from build123d import *

# Parameters (mm, degrees)
PAD_DEPTH             = 24
POCKET_DEPTH          = 3
SKETCH002_W           = 70
SKETCH002_H           = 18.5
POCKET001_DEPTH       = 18
POLARPATTERN_COUNT    = 3
POCKET002_DEPTH       = 6
CHAMFER_SIZE          = 8
FILLET_R              = 13
FILLET001_R           = 11
CHAMFER001_SIZE       = 16.1
FILLET002_R           = 11
FILLET003_R           = 12
POCKET003_DEPTH       = 6
POCKET004_DEPTH       = 18
POCKET005_DEPTH       = 21.001
SKETCH007_W           = 15.5
SKETCH007_H           = 15
POCKET006_DEPTH       = 5
SKETCH010_W           = 13.6
SKETCH010_H           = 9
POCKET009_DEPTH       = 15.5
POCKET010_DEPTH       = 3
SKETCH012_R           = 1.85
SKETCH012_R_2         = 0.99
POCKET011_DEPTH       = 498.0492855781
POLARPATTERN001_COUNT = 3
POCKET012_DEPTH       = 12


with BuildPart() as part:
    # Sketch → Pad (new body)
    with BuildSketch(Plane.XY):
        Polygon((0, 112.2094915052), (-97.1762701892, -56.1047457526), (97.1762701892, -56.1047457526), align=None)
        Polygon((0, 62.2094915052), (-53.875, -31.1047457526), (53.875, -31.1047457526), align=None, mode=Mode.SUBTRACT)
    extrude(amount=PAD_DEPTH)

    # Sketch001 (on Face8 of Pad) → Pocket (cut)
    with BuildSketch(Plane.XY.offset(24)):
        Polygon((0, 98.2094915052), (-85.0519145362, -49.1047457526), (85.0519145362, -49.1047457526), align=None)
        Polygon((0, 76.2094915052), (-65.999355653, -38.1047457526), (65.999355653, -38.1047457526), align=None, mode=Mode.SUBTRACT)
    extrude(amount=-POCKET_DEPTH, mode=Mode.SUBTRACT)

    # Sketch002 (on Face4 of Pocket) → Pocket001 (cut)
    with BuildSketch(Plane(origin=(0, 0, 0), x_dir=(1, 0, 0), z_dir=(0, 0, -1))):
        with Locations((0, 43.6047457526)):
            Rectangle(SKETCH002_W, SKETCH002_H)
    pocket001 = extrude(amount=-POCKET001_DEPTH, mode=Mode.SUBTRACT)

    # PolarPattern: Pocket001 ×3 about axis
    polarpattern_axis = Axis((0, 0, 0), (0, 0, -1))
    for i in range(1, POLARPATTERN_COUNT):
        add(pocket001.rotate(polarpattern_axis, i * 360 / POLARPATTERN_COUNT), mode=Mode.SUBTRACT)

    # Sketch003 (on Face4 of PolarPattern) → Pocket002 (cut)
    with BuildSketch(Plane(origin=(0, 0, 0), x_dir=(1, 0, 0), z_dir=(0, 0, -1))):
        Polygon((0, -100.2094915052), (86.7839653438, 50.1047457526), (-86.7839653438, 50.1047457526), align=None)
        Polygon((0, -74.2094915052), (64.2673048454, 37.1047457526), (-64.2673048454, 37.1047457526), align=None, mode=Mode.SUBTRACT)
    extrude(amount=-POCKET002_DEPTH, mode=Mode.SUBTRACT)

    # Chamfer
    chamfer_edges = [part.edges().sort_by_distance(p)[0] for p in [
        (-53.875, -31.104746, 12),
        (53.875, -31.104746, 12),
        (0, 62.209492, 12),
    ]]
    chamfer(chamfer_edges, length=CHAMFER_SIZE)

    # Fillet
    fillet_edges = [part.edges().sort_by_distance(p)[0] for p in [
        (0, 100.209492, 3),
        (-86.783965, -50.104746, 3),
        (86.783965, -50.104746, 3),
    ]]
    fillet(fillet_edges, radius=FILLET_R)

    # Fillet001
    fillet001_edges = [part.edges().sort_by_distance(p)[0] for p in [
        (0, 74.209492, 3),
        (64.267305, -37.104746, 3),
        (-64.267305, -37.104746, 3),
    ]]
    fillet(fillet001_edges, radius=FILLET001_R)

    # Chamfer001
    chamfer001_edges = [part.edges().sort_by_distance(p)[0] for p in [
        (97.17627, -56.104746, 12),
        (0, 112.209492, 12),
        (-97.17627, -56.104746, 12),
    ]]
    chamfer(chamfer001_edges, length=CHAMFER001_SIZE)

    # Fillet002
    fillet002_edges = [part.edges().sort_by_distance(p)[0] for p in [
        (0, 98.209492, 22.5),
        (-85.051915, -49.104746, 22.5),
        (85.051915, -49.104746, 22.5),
    ]]
    fillet(fillet002_edges, radius=FILLET002_R)

    # Fillet003
    fillet003_edges = [part.edges().sort_by_distance(p)[0] for p in [
        (65.999356, -38.104746, 22.5),
        (0, 76.209492, 22.5),
        (-65.999356, -38.104746, 22.5),
    ]]
    fillet(fillet003_edges, radius=FILLET003_R)

    # Sketch004 (on Face60 of Fillet003) → Pocket003 (cut)
    with BuildSketch(Plane(origin=(0, 0, 6), x_dir=(1, 0, 0), z_dir=(0, 0, -1))):
        Polygon((-8.75, -71.2664825043), (8.75, -71.2664825043), (8.75, -94.7664825043), (4, -94.7664825043), (4, -98.2664825043), (-4, -98.2664825043), (-4, -94.7664825043), (-8.75, -94.7664825043), align=None)
    extrude(amount=-POCKET003_DEPTH, mode=Mode.SUBTRACT)

    # Sketch005 (on Face29 of Pocket003) → Pocket004 (cut)
    with BuildSketch(Plane(origin=(0, 0, 0), x_dir=(1, 0, 0), z_dir=(0, 0, -1))):
        Polygon((46.1715988394, 38.9547457526), (68.6882593378, 51.9547457526), (79.3382593378, 33.508404652), (56.8215988394, 20.508404652), align=None)
    extrude(amount=-POCKET004_DEPTH, mode=Mode.SUBTRACT)

    # Sketch006 (on Face1 of Pocket004) → Pocket005 (cut, through all)
    with BuildSketch(Plane.XY.offset(21)):
        with BuildLine():
            ThreePointArc((1.5, 85.0404521425), (0, 86.5404521425), (-1.5, 85.0404521425))
            Line((-1.5, 85.0404521425), (-1.5, 66.0404521425))
            ThreePointArc((-1.5, 66.0404521425), (0, 64.5404521425), (1.5, 66.0404521425))
            Line((1.5, 85.0404521425), (1.5, 66.0404521425))
        make_face()
    extrude(amount=-POCKET005_DEPTH, mode=Mode.SUBTRACT)

    # Sketch007 (on Face24 of Pocket005) → Pocket006 (cut)
    with BuildSketch(Plane(origin=(-48.5881350946, 28.0523728763, 0), x_dir=(-0.5, -0.8660254038, 0), z_dir=(-0.8660254038, 0.5, 0))):
        with Locations((-47.3262701892, 13.5)):
            Rectangle(SKETCH007_W, SKETCH007_H)
    extrude(amount=-POCKET006_DEPTH, mode=Mode.SUBTRACT)

    # Sketch010 (on Face79 of Pocket006) → Pocket009 (cut)
    with BuildSketch(Plane(origin=(-44.2580080757, 25.5523728763, 0), x_dir=(-0.5, -0.8660254038, 0), z_dir=(-0.8660254038, 0.5, 0))):
        with Locations((-47.3262701892, 13.5)):
            Rectangle(SKETCH010_W, SKETCH010_H)
    extrude(amount=-POCKET009_DEPTH, mode=Mode.SUBTRACT)

    # Sketch011 (on Face21 of Pocket009) → Pocket010 (cut)
    with BuildSketch(Plane(origin=(0, 0, 6), x_dir=(1, 0, 0), z_dir=(0, 0, -1))):
        Polygon((-21.0413798427, -59.7570681827), (-11.6817654684, -54.3532923042), (-6.658482036, -63.0538744299), (-16.0180964103, -68.4576503084), align=None)
    extrude(amount=-POCKET010_DEPTH, mode=Mode.SUBTRACT)

    # Sketch012 (on Face54 of Pocket010) → Pocket011 (cut, through all)
    with BuildSketch(Plane(origin=(0, 0, 0), x_dir=(1, 0, 0), z_dir=(0, 0, -1))):
        with Locations((-13.5, -82.7032108255)):
            Circle(SKETCH012_R)
        with Locations((13.5, -82.7032108255)):
            Circle(SKETCH012_R)
        with Locations((-6.25, -96.5164825043)):
            Circle(SKETCH012_R_2)
        with Locations((6.25, -96.5164825043)):
            Circle(SKETCH012_R_2)
        with Locations((-27.2463245869, -59.0174730012)):
            Circle(SKETCH012_R_2)
        with Locations((-47.1862074814, -27.2405827309)):
            Circle(SKETCH012_R_2)
        with Locations((-64.7337931796, 5.9127272486)):
            Circle(SKETCH012_R_2)
        with Locations((-10.791841915, -49.5174730012)):
            Circle(SKETCH012_R_2)
        with Locations((-28.3394276132, -16.3641630217)):
            Circle(SKETCH012_R_2)
        with Locations((-48.2793105078, 15.4127272487)):
            Circle(SKETCH012_R_2)
    pocket011 = extrude(amount=-POCKET011_DEPTH, mode=Mode.SUBTRACT)

    # PolarPattern001: Pocket011 ×3 about axis
    polarpattern001_axis = Axis((0, 0, 0), (0, 0, -1))
    for i in range(1, POLARPATTERN001_COUNT):
        add(pocket011.rotate(polarpattern001_axis, i * 360 / POLARPATTERN001_COUNT), mode=Mode.SUBTRACT)

    # Sketch013 (on Face132 of PolarPattern001) → Pocket012 (cut)
    with BuildSketch(Plane(origin=(0, 0, 6), x_dir=(1, 0, 0), z_dir=(0, 0, -1))):
        Polygon((58.553649647, 21.508404652), (63.3167893678, 24.258404652), (66.3167893678, 19.0622522293), (61.553649647, 16.3122522293), align=None)
    extrude(amount=-POCKET012_DEPTH, mode=Mode.SUBTRACT)


solid = part.part
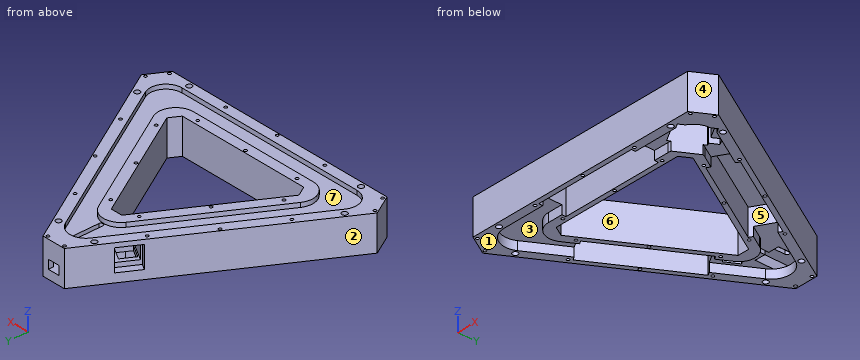
Source: CAD feature listing. Evaluate the final solid. Frame: model axes, mm. Face numbers are marked on the shaded views. A direction names the side the tool comes from. Coordinates: 2 decimals unless noted, no trailing zeros.
Item 1: Pull-direction query (Y, two-part tool) for the marked faces 1, 2, 3 and 4; classes: pulls with the +Y half, pulls with the -Y half, needs draft (parallel to the pull), parting line crosses it, or undercut.
Output values:
face 1: needs draft
face 2: pulls with the +Y half
face 3: undercut
face 4: pulls with the -Y half
Item 2: First-contact query: P1, Ø1.8, axis at x = 37.49, y = -53.1, coming from the +Z side; P2, Ø6.5, axis at y = 87.5, z = 10, coming from the +X side; P3, Ø1, axis at x = 25.5, z = 16.5, coming from the +Y side; P4, Ø6, axis at y = 77, z = 12, coming from the -X side. Flat tips, straight axial feed; report the tip coordinate or a pass-through.
Output values:
P1: passes through
P2: stops at x = 16.14
P3: stops at y = 68.91
P4: stops at x = -21.05
Item 3: Cut plane A-A (z = 2.75). Count the separate pieces of the cut face and the enclosed holes in it, plus the area to 3 significant figures.
Output values:
separate pieces: 2
enclosed holes: 32
area: 3,930 mm2
Item 4: Set-up query: the marked faces 5, 6 and 7. Return all of +Z, -Z, +X, -X, +Y, -Y with unobstructed straight access to the full face (end or side cutting, diameter ignored); none if empty.
Output values:
face 5: -Z
face 6: +Z, -Z
face 7: +Z
Item 5: Material intervals for line 1 (X direction, y = -18.5, z = 21.5); line 2 (X direction, y = -26.5, z = 15); line 3 (Y direction, x = -26, z = 1), sorted ascending.
Output values:
line 1: x = -75.47 to -67.38, -54.68 to -46.6, 46.6 to 54.68, 67.38 to 75.47
line 2: x = -80.08 to -48.53, 48.53 to 53.36, 67.2 to 80.08
line 3: y = -56.1 to -52.85, -34.35 to -31.1, 17.18 to 23.68, 55.43 to 67.18
